Here's how the part is built. I have some questions about the finished solid (model axes, mm). A direction names the side the tool comes from. Round coordinates to 2 decimals unless told otherwise and drop trailing zeros. Write each loop counter-clockwise with the first axis right and the second up, starting at its lowest first coordinate (ties: lowest second). Pieces come first, ordered by that corner, then holes. Notation, with made-up numbers: (63.5, 19) -> (100.5, 19) arc R17 cw to (100.5, 49) -> close; hole circle Ø4 at (-0.5, 59). An arc over 180 degrees is marked (long way). Answer as CSV lines item,"result".
```python
from build123d import *

# Parameters (mm, degrees)
F2_DEPTH = 19.05
F3_DEPTH = 19.051
F4_R     = 10.16
F5_R     = 10.16


with BuildPart() as f2:
    # F0 (on Front) → F2 (new body)
    with BuildSketch(Plane.XZ):
        Polygon((0, 95.157677), (-25.4, 95.157677), (-25.4, -31.842323), (69.85, -31.842323), (69.85, -6.442323), align=None)
    extrude(amount=-F2_DEPTH)

    # F1 (on face) → F3 (cut, through all)
    with BuildSketch(Plane.XZ):
        Polygon((51.097869, -12.792323), (-6.35, 70.768214), (-6.35, -12.792323), align=None)
    extrude(amount=-F3_DEPTH, mode=Mode.SUBTRACT)

    # F4
    f4_edges = [f2.edges().sort_by_distance(p)[0] for p in [
        (-6.35, 9.525, -12.792323),
        (51.097869, 9.525, -12.792323),
    ]]
    fillet(f4_edges, radius=F4_R)

    # F5
    f5_edges = [f2.edges().sort_by_distance(p)[0] for p in [
        (-6.35, 9.525, 70.768214),
    ]]
    fillet(f5_edges, radius=F5_R)


solid = f2.part
```
1. Suppose I cut it at B-B on z = 41. Please give me the cut outline in (x, y), and give its area (3 significant figures).
Numbers:
outline,"(-25.4, 0) -> (-5.91, 0) -> (-5.91, 19.05) -> (-25.4, 19.05) -> close; (14.12, 0) -> (37.23, 0) -> (37.23, 19.05) -> (14.12, 19.05) -> close"
area,"812 mm^2"
2. Suppose I cut it at D-D on z = 63. Please give me the cut outline in (x, y), and give its area (3 significant figures).
Numbers:
outline,"(-25.4, 0) -> (22.11, 0) -> (22.11, 19.05) -> (-25.4, 19.05) -> close"
area,"905 mm^2"
3. Suppose I cut it at C-C on x = -3. Please give me the cut outline in (y, z).
Numbers:
outline,"(0, -31.84) -> (19.05, -31.84) -> (19.05, -10.17) -> (0, -10.17) -> close; (0, 45.6) -> (19.05, 45.6) -> (19.05, 95.16) -> (0, 95.16) -> close"
4. If we mould it in two halves opening along Z, with no side actions, what happens to faces 3 (the face through (-13, 9, 95.158)), 4 (the face through (40.85, 9.66, -7.22)), 5 (the face through (22, 19.05, 33))? For each: released by +Z, released by -Z, zero draft, split by the parting line, or undercut.
Numbers:
face 3,"released by +Z"
face 4,"undercut"
face 5,"zero draft"
5. If I drill on line 1 (Z direction, x = 26.5, y = 14); line 2 (Z direction, x = 22, y = 18); line 3 (X direction, y = 5.25, z = 4), over which ranges is the centre line in solid material (lowest first)?
Numbers:
line 1,"z = -31.84 to -12.79, 22.99 to 56.61"
line 2,"z = -31.84 to -12.79, 29.53 to 63.16"
line 3,"x = -25.4 to -6.35, 39.55 to 62.67"
6. On a 3-axis mill with a long thin cutter (end or side, diameter ignored), from which of +Z, -Z, +X, -X, +Y, -Y can I reach the whole of each face in a straight line? I mean faces 1 (the face through (0.97, 9.66, 47.81)), 2 (the face through (22, 9, -31.842)). Say none if no direction works.
Numbers:
face 1,"+Y, -Y"
face 2,"-Z, +X, -X, +Y, -Y"
7. For pin 1 Ø9.5 at (x, y) = (11, 12.5) entering from +Z; pin 2 Ø5.5 at (y, z) = (9.5, 11) entering from +X; pin 3 Ø8 at (y, z) = (5, 6.5) entering from +X, each with a flat end and sliding along its axis, tell me the tip position at first contact or that it passes through.
Numbers:
pin 1,"stops at z = 86.07"
pin 2,"stops at x = 59.75"
pin 3,"stops at x = 63.7"
8. Suppose I cut it at A-A on y = 12.25. Please give me the cut outline in (x, z), and give its area (3 significant figures).
Numbers:
outline,"(-25.4, -31.84) -> (69.85, -31.84) -> (69.85, -6.44) -> (0, 95.16) -> (-25.4, 95.16) -> close; hole (-6.35, -2.63) arc R10.16 ccw to (3.81, -12.79) -> (31.78, -12.79) arc R10.16 ccw to (40.16, 3.12) -> (12.18, 43.81) arc R10.16 ccw to (-6.35, 38.06) -> close"
area,"6,460 mm^2"
